Autodesk Fusion 360 part; units mm, degrees
sketch "Sketch1" plane through (0, 0, 0) normal (0, 0, 1) x (1, 0, 0)
  line L0 (110, -92.5) -> (-110, -92.5)
  line L1 (-110, -92.5) -> (-110, 92.5)
  line L2 (-110, 92.5) -> (110, 92.5)
  line L3 (110, 92.5) -> (110, -92.5)
  line L4 (110, -92.5) -> (-110, 92.5) construction
  line L5 (-110, -92.5) -> (110, 92.5) construction
  line L6 (-110, 92.5) -> (97.5144, 92.5)
  line L7 (-53.7181, -92.5) -> (-110, -92.5)
  line L8 (-110, -92.5) -> (-110, 92.5)
  line L9 (-50, 92.5) -> (-45, 92.5)
  line L10 (-45, 92.5) -> (-45, -92.5)
  line L11 (-45, -92.5) -> (-50, -92.5)
  line L12 (-50, -92.5) -> (-50, 92.5)
  line L13 (10, 92.5) -> (15, 92.5)
  line L14 (15, 92.5) -> (15, -92.5)
  line L15 (15, -92.5) -> (10, -92.5)
  line L16 (10, -92.5) -> (10, 92.5)
  line L17 (70, 92.5) -> (75, 92.5)
  line L18 (75, 92.5) -> (75, -92.5)
  line L19 (75, -92.5) -> (70, -92.5)
  line L20 (70, -92.5) -> (70, 92.5)
  line L21 (75, 42.0875) -> (75, 63.0682)
  line L22 (-110, 68) -> (-110, 42.0875)
  line L23 (75, -17.4811) -> (75, -23.4712)
  line L24 (-110, -23.4712) -> (-110, -17.4811)
  line L25 (-110, 32.5) -> (75, 32.5)
  line L26 (75, 32.5) -> (75, 27.5)
  line L27 (75, 27.5) -> (-110, 27.5)
  line L28 (-110, 27.5) -> (-110, 32.5)
  line L29 (-110, -27.5) -> (75, -27.5)
  line L30 (75, -27.5) -> (75, -32.5)
  line L31 (75, -32.5) -> (-110, -32.5)
  line L32 (-110, -32.5) -> (-110, -27.5)
  line L33 (-110, -87.5) -> (75, -87.5)
  line L34 (75, -87.5) -> (75, -92.5)
  line L35 (75, -92.5) -> (-110, -92.5)
  line L36 (-110, -92.5) -> (-110, -87.5)
  line L37 (-110, 92.5) -> (75, 92.5)
  line L38 (75, 92.5) -> (75, 87.5)
  line L39 (75, 87.5) -> (-110, 87.5)
  line L40 (-110, 87.5) -> (-110, 92.5)
  line L41 (-110, 92.5) -> (-105, 92.5)
  line L42 (-105, 92.5) -> (-105, -92.5)
  line L43 (-105, -92.5) -> (-110, -92.5)
  line L44 (-110, -92.5) -> (-110, 92.5)
  line L45 (75, 37.5) -> (110, 37.5) construction
  line L46 (75, -37.5) -> (110, -37.5) construction
  circle A0 centre (76.8705, -4.3263) radius 25 construction
  circle A1 centre (78.6242, -22.2407) radius 1.75
  circle A2 centre (76.6017, 13.6717) radius 1.75
  line L47 (75, 25.3235) -> (110, 25.3235) construction
  dimension "d3" = 220
  dimension "d5" = 5
  dimension "d6" = 5
  dimension "d8" = 5
  dimension "d10" = 55
  dimension "d11" = 55
  dimension "d13" = 5
  dimension "d16" = 5
  dimension "d17" = 5
  dimension "d18" = 5
  dimension "d19" = 55
  dimension "d20" = 55
  dimension "d22" = 55
  dimension "d23" = 5
  dimension "d24" = 55
  dimension "d25" = 55
  dimension "d26" = 55
  dimension "d27" = 50
  dimension "d32" = 3.5
  dimension "d33" = 3.5
  dimension "d34" = 18
  dimension "d35" = 18
extrude "Extrude7" add sketch "Sketch1" along normal blind 5 contours L0 L18 L19 L20 L33 L34 L35 | L0 L14 L20 L33 L35 | L18 L20 L31 L33 | L0 L14 L15 L16 L33 L35 | L18 L20 L29 L30 L31 | L2 L6 L17 L18 L20 L37 L38 L39 | L0 L10 L16 L33 L35 | L14 L16 L31 L33 | L14 L20 L29 L31 | L18 L20 L23 L27 L29 A2 | L2 L6 L14 L20 L37 L39 | L18 L20 L21 L25 L39 | L0 L10 L11 L12 L33 L35 | L14 L16 L29 L31 | L2 L6 L13 L14 L16 L37 L39 | L0 L7 L12 L33 L35 L42 | L10 L12 L31 L33 | L10 L16 L29 L31 | L14 L16 L27 L29 | L14 L20 L25 L27 | L18 L20 L25 L26 L27 | L2 L6 L10 L16 L37 L39 | L14 L16 L25 L39 | L10 L12 L29 L31 | L14 L16 L25 L27 | L18 A2 | L2 L6 L9 L10 L12 L37 L39 | L0 L1 L7 L8 L33 L35 L36 L42 L43 L44 | L12 L29 L31 L42 | L1 L8 L31 L33 L42 L44 | L10 L12 L27 L29 | L10 L16 L25 L27 | L2 L6 L12 L37 L39 L42 | L10 L12 L25 L39 | L1 L8 L29 L31 L32 L42 L44 | L10 L12 L25 L27 | L1 L2 L6 L8 L37 L39 L40 L41 L42 L44 | L12 L25 L27 L42 | L1 L8 L24 L27 L29 L42 L44 | L1 L8 L22 L25 L39 L42 L44 | L1 L8 L25 L27 L28 L42 L44 picked at (74.9727, 13.8309)
sketch "Sketch5" plane through (0, 0, 0) normal (0, 0, 1) x (1, 0, 0)
  line L0 (-110, 92.5) -> (-105, 87.5) construction
  line L1 (-105, 92.5) -> (-110, 87.5) construction
  circle A0 centre (-107.5, 90) radius 1.4
  line L2 (70, 92.5) -> (75, 87.5) construction
  line L3 (75, 92.5) -> (70, 87.5) construction
  circle A1 centre (72.5, 90) radius 1.4
  line L4 (70, -87.5) -> (75, -92.5) construction
  line L5 (75, -87.5) -> (70, -92.5) construction
  circle A2 centre (72.5, -90) radius 1.4
  line L6 (-110, -87.5) -> (-105, -92.5) construction
  line L7 (-105, -87.5) -> (-110, -92.5) construction
  circle A3 centre (-107.5, -90) radius 1.4
  dimension "d54" = 2.8
  dimension "d55" = 2.8
  dimension "d56" = 2.8
  dimension "d57" = 2.8
extrude "Extrude8" cut sketch "Sketch5" along normal through all
equation "Board_piece_lenght = 40 mm"
equation "d5 = Wall_width"
equation "d6 = Wall_width"
equation "Wall_width = 5 mm"
equation "d8 = Wall_width"
equation "d10 = Inner_sqauare"
equation "d11 = Inner_sqauare"
equation "Inner_sqauare = 55 mm"
equation "d13 = Wall_width"
equation "d16 = Wall_width"
equation "d17 = Wall_width"
equation "d18 = Wall_width"
equation "d19 = Inner_sqauare"
equation "d20 = Inner_sqauare"
equation "d22 = Inner_sqauare"
equation "d23 = Wall_width"
equation "d24 = Inner_sqauare"
equation "d25 = Inner_sqauare"
equation "d26 = Inner_sqauare"
Could you check a few things on this model? Use its own coordinates, in mm. Give positions to 0.01 mm unless a question says otherwise; leave off trailing zeros. Order: outer loops, then holes, each group sorted by start corner. A loop starts at its lowest first (then second) coordinate and runs counter-clockwise, first axis right, second up. Notation, with made-up numbers: (-10.5, 37) - (35.5, 37) arc R25 ccw to (35.5, 64) - close; hole circle Ø9 at (46.5, 1.5). An arc over 180 degrees is marked (long way). One line per item, written item: value. Start each with the question number.
1. Imagine slicing it at B-B on x = 34.5. List the corners of the cut face in (y, z) for me.
2. For P1, Ø6, axis at x = 5.5, y = -74, coming from the -Z side, with a flat end and sliding along its axis, tell me the tip position at first contact or that it passes through.
3. If I drill on probe 1 along Y at (x, z) = (-58, 2); probe 2 along Y at (x, z) = (-107.5, 2.9); probe 3 along X at (y, z) = (-63, 1.05), over which ranges is the centre line in solid material (lowest first)?
4. Imagine slicing it at C-C on z = 3.5. Give the number of separate pieces and of enclosed holes in the cut face, plus the area to 3 significant figures.
5. Imagine slicing it at A-A on y = -3. List the corners of the cut face in (x, z) for me.
Values:
1. outline: (-92.5, 0) - (-87.5, 0) - (-87.5, 5) - (-92.5, 5) - close; (-32.5, 0) - (-27.5, 0) - (-27.5, 5) - (-32.5, 5) - close; (27.5, 0) - (32.5, 0) - (32.5, 5) - (27.5, 5) - close; (87.5, 0) - (92.5, 0) - (92.5, 5) - (87.5, 5) - close
2. P1: through
3. probe 1: -92.5 to -87.5, -32.5 to -27.5, 27.5 to 32.5, 87.5 to 92.5
3. probe 2: -92.5 to -91.4, -88.6 to 88.6, 91.4 to 92.5
3. probe 3: -110 to -105, -50 to -45, 10 to 15, 70 to 75
4. separate pieces: 1
4. enclosed holes: 13
4. area: 6,980 mm²
5. outline: (-110, 0) - (-105, 0) - (-105, 5) - (-110, 5) - close; (-50, 0) - (-45, 0) - (-45, 5) - (-50, 5) - close; (10, 0) - (15, 0) - (15, 5) - (10, 5) - close; (70, 0) - (75, 0) - (75, 5) - (70, 5) - close
